For this review, use the dimensioned drawing (mm, ordinates from the lowest corner) and the shaded views. Round coordinates to 2 decimals unless told otherwise and drop trailing zeros. Order: outer loops, then holes, each group sorted by start corner. A loop starts at its lowest first (then second) coordinate and runs counter-clockwise, first axis right, second up. Notation, with made-up numbers: (32.25, 2) - (55.25, 2) arc R29 ccw to (55.25, 29) - close; hole circle Ø2 at (-18, -22). An arc over 180 degrees is marked (long way). Write each question's results on one line, items separated by ' | '. Start each with the question number.
(1) For L1, parallel to X at y = 80, z = 0.95 (1 decimal); L2, parallel to X at y = 66.5, z = 4.6 (1 decimal); L3, parallel to Y at x = 55.5, z = 4.7 (1 decimal), list the stretches that pass through material, from the lowest coordinate up. Write a range as from..to.
(2) Take a section at B-B, the plane z = 2.1. Give the boundary of the cut face in (x, y) (1 decimal).
(3) Take a section at C-C, the plane y = 32.5. Give the boundary of the cut face in (x, z).
(4) Insertion check: pin 1 Ø3 at (y, z) = (80.5, 2) entering from +X; pin 2 Ø1.7 at (x, z) = (90, 2) entering from -Y; pin 3 Ø1.7 at (y, z) = (3.5, 2) entering from -X; pin 4 Ø9.5 at (x, y) = (15.31, 70.28) entering from -Z. Each pin has a flat end and moves straight along its axis. Give the tip position at first contact, or say it passes through.
(5) Take a section at D-D, the plane x = 32.5. Give the boundary of the cut face in (y, z).
(6) Take a section at A-A, the plane x = 97. Give the boundary of the cut face in (y, z).
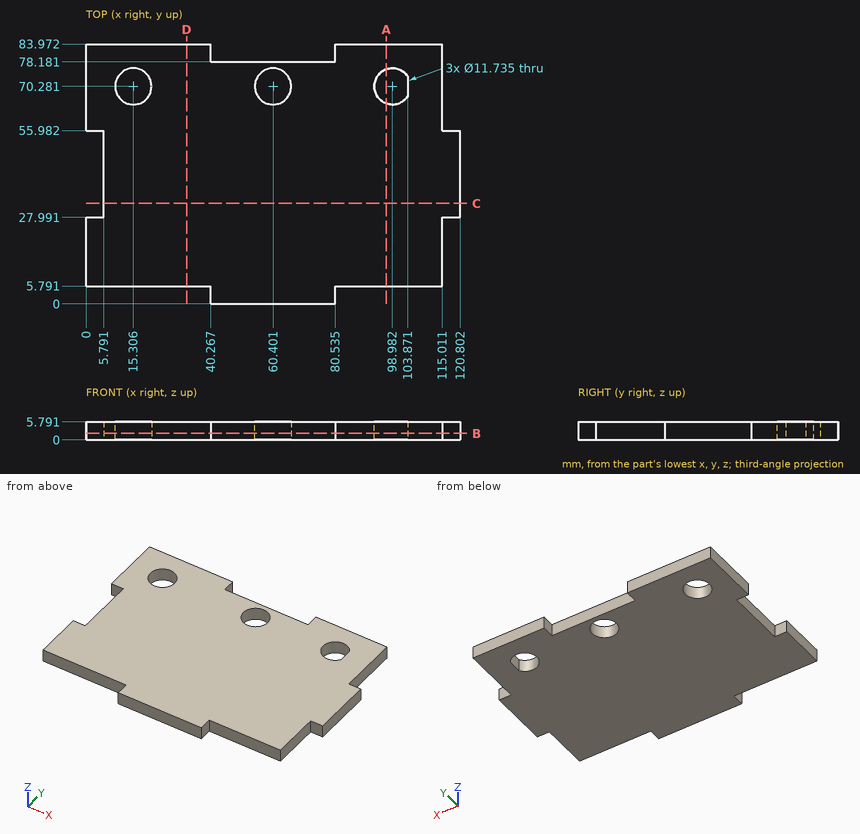
Results below:
1) L1: x = 0..40.3, 80.5..115 | L2: x = 0..10.8, 19.8..55.9, 64.9..94.5, 103.5..115 | L3: y = 0..67.1, 73.5..78.2
2) outline: (0, 5.8) - (40.3, 5.8) - (40.3, 0) - (80.5, 0) - (80.5, 5.8) - (115, 5.8) - (115, 28) - (120.8, 28) - (120.8, 56) - (115, 56) - (115, 84) - (80.5, 84) - (80.5, 78.2) - (40.3, 78.2) - (40.3, 84) - (0, 84) - (0, 56) - (5.8, 56) - (5.8, 28) - (0, 28) - close; hole circle Ø11.7 at (15.3, 70.3); hole circle Ø11.7 at (60.4, 70.3); hole (103.9, 67) - (103.9, 73.5) arc R5.9 ccw (long way) to start
3) outline: (5.79, 0) - (120.8, 0) - (120.8, 5.79) - (5.79, 5.79) - close
4) pin 1: stops at x = 115.01 | pin 2: stops at y = 5.79 | pin 3: stops at x = 40.27 | pin 4: passes through
5) outline: (5.79, 0) - (83.97, 0) - (83.97, 5.79) - (5.79, 5.79) - close
6) outline: (5.79, 0) - (64.76, 0) - (64.76, 5.79) - (5.79, 5.79) - close; (75.8, 0) - (83.97, 0) - (83.97, 5.79) - (75.8, 5.79) - close
